```python
from build123d import *

# Parameters (mm, degrees)
F1_DEPTH = 60


with BuildPart() as f1:
    # F0 (on Top) → F1 (new body)
    with BuildSketch(Plane.XY):
        with BuildLine():
            Line((0, -41.300625), (23.163913, -41.300625))
            ThreePointArc((23.163913, -41.300625), (37.541736, -10.033364), (14.019156, 15.087376))
            ThreePointArc((14.019156, 15.087376), (24.581036, 33.266488), (7.719544, 45.825291))
            Line((7.719544, 45.825291), (7.719544, 64.319231))
            ThreePointArc((7.719544, 64.319231), (-1.807018, 59.74027), (-11.333581, 64.319231))
            Line((-11.333581, 64.319231), (-11.333581, 45.825291))
            ThreePointArc((-11.333581, 45.825291), (-23.6358, 30.608301), (-14.024769, 13.563377))
            ThreePointArc((-14.024769, 13.563377), (-29.434517, -15.124752), (-10.062043, -41.300625))
            Line((-10.062043, -41.300625), (0, -41.300625))
        make_face()
    extrude(amount=F1_DEPTH)


solid = f1.part
```
For this review, take the finished solid that the model builds, in its own axes (mm). A direction names the side the tool comes from. Coordinates: 2 decimals unless noted, no trailing zeros. Order: outer loops, then holes, each group sorted by start corner. A loop starts at its lowest first (then second) coordinate and runs counter-clockwise, first axis right, second up. Notation, with made-up numbers: (58.25, -14.75) -> (78.25, -14.75) arc R33 cw to (78.25, 24.25) -> close; hole circle Ø8 at (35.5, 12). An arc over 180 degrees is marked (long way). Answer as CSV lines item,"result".
Q1. Wall thickness on line 1 along Y through (x, z) = (22.5, 28); line 2 along Y through (x, z) = (-18, 56); line 3 along Y through (x, z) = (-1, 37): over which ranges is each line inside the solid? List them lowest first. Write a range as [from, to].
Model answer:
line 1,"y = [-41.3, 11.75], [21.72, 38.47]"
line 2,"y = [-36.76, 10.89], [16.28, 42.04]"
line 3,"y = [-41.3, 59.77]"
Q2. For faces 1 (the face through (-11.334, 55, 30)), 2 (the face through (6, -41.301, 30)), list the 3-axis set-ups (+Z, -Z, +X, -X, +Y, -Y) from which the entire face can be reached by the end or side of a thin tool; tool diameter is ignored.
Model answer:
face 1,"+Z, -Z, -X, +Y"
face 2,"+Z, -Z, +X, -X, -Y"
Q3. We need section B-B (z = 39). State the section outline as (x, y) points, plus the area to 3 significant figures.
Model answer:
outline,"(-14.02, 13.56) arc R30.41 ccw to (-10.06, -41.3) -> (23.16, -41.3) arc R30.85 ccw to (14.02, 15.09) arc R15.79 ccw to (7.72, 45.83) -> (7.72, 64.32) arc R12.2 cw to (-11.33, 64.32) -> (-11.33, 45.83) arc R17.41 ccw to start"
area,"4,820 mm2"
Q4. We need section D-D (x = 28). State the section outline as (y, z) points, plus the area to 3 significant figures.
Model answer:
outline,"(-37.65, 0) -> (7.71, 0) -> (7.71, 60) -> (-37.65, 60) -> close"
area,"2,720 mm2"
Q5. We need section C-C (y = 55.5). State the section outline as (x, z) points.
Model answer:
outline,"(-11.33, 0) -> (7.72, 0) -> (7.72, 60) -> (-11.33, 60) -> close"
Q6. Draft analysis for pull direction Y (two halves, no side actions). For faces 3 (the face through (-1.65, 59.74, 29.58)), 4 (the face through (4, 1, 0)), 5 (the face through (24.642, 32.95, 29.58)), state which applies: released by +Y, released by -Y, zero draft, split by the parting line, or undercut.
Model answer:
face 3,"released by +Y"
face 4,"zero draft"
face 5,"undercut"
Q7. We need section A-A (x = -22.5). State the section outline as (y, z) points.
Model answer:
outline,"(-32.36, 0) -> (6.49, 0) -> (6.49, 60) -> (-32.36, 60) -> close; (22.82, 0) -> (35.5, 0) -> (35.5, 60) -> (22.82, 60) -> close"
Q8. Clearance check with flat-ended pins moving along their axes: pin 1 Ø3 at (y, z) = (12.5, 30.5) entering from -X; pin 2 Ø8 at (y, z) = (2, 50.5) entering from +X; pin 3 Ø6 at (x, y) = (-22.5, 12.5) entering from -Z; pin 4 Ø5.5 at (y, z) = (56, 19.5) entering from +X. State where each tip first meets the part, or that it passes through.
Model answer:
pin 1,"stops at x = -17.86"
pin 2,"stops at x = 35.08"
pin 3,"passes through"
pin 4,"stops at x = 7.72"
